The model under review builds one solid part; all positions refer to its coordinate system, in mm. A direction names the side the tool comes from. Round coordinates to 2 decimals unless told otherwise and drop trailing zeros. Write each loop counter-clockwise with the first axis right and the second up, starting at its lowest first coordinate (ties: lowest second). Pieces come first, ordered by that corner, then holes. Notation, with made-up numbers: (65.5, 20) -> (70.5, 20) arc R17 ccw to (70.5, 27) -> close; hole circle Ø2 at (70.25, 18.5). An arc over 180 degrees is marked (long way). Answer as a JSON object with one key per item and string values. Group by question number.
1) We need section A-A, the plane y = 11.5. Write out the cut boundary in (x, z) (1 decimal).
2) Machinability: for faces 1 (the flat face through (4, 0, 0)), 2 (the flat face through (-4, 17.78, 0)), 3 (the cylindrical face through (-8.68, 29.77, 1.93)), which of the approach directions +Z, -Z, +X, -X, +Y, -Y give a long, thin tool a straight path to every point of the face, cutting with its end or side? Answer none if there is none.
3) We need section C-C, the plane x = 4. Write out the cut boundary in (y, z) (3 decimals).
4) We need section B-B, the plane z = 6.5. Write out the cut boundary in (x, y) (3 decimals).
5) Mouldability with a two-part tool opening along X and no side actions: class faces 4 (the cylindrical face through (0.708, 28.486, 3.186)), 5 (the cylindrical face through (7.5, 15, -8.2)), 6 (the flat face through (9.1, 24.765, 0.1)) as pulls with the +X half, pulls with the -X half, needs draft (parallel to the pull), parting line crosses it, or undercut.
6) We need section D-D, the plane x = -8. Write out the cut boundary in (y, z) (3 decimals), then the cut area to 3 significant figures.
7) To check wall thickness, follow probe 1 along Y at (x, z) = (4, 0) (3 decimals); probe 2 along Y at (x, z) = (-6.5, -7.5) (3 decimals); probe 3 along Z at (x, y) = (5.5, 8.89). State the ranges of each line that lie inside material, in increasing order. Write a range as [from, to].
8) Insertion check: pin 1 Ø1.5 at (y, z) = (4.5, -9) entering from +X; pin 2 Ø8 at (y, z) = (6, 3.5) entering from +X; pin 3 Ø2 at (y, z) = (28, -1.5) entering from +X. Each pin has a flat end and moves straight along its axis. Give the tip position at first contact, or say it passes through.
from build123d import *

# Parameters (mm, degrees)
CROQUIS1_R                     = 11.1125
SALIENTE_EXTRUIR1_DEPTH        = 34.925
CORTAR_EXTRUIR2_START          = 10.16
CROQUIS12_R                    = 11.1125
CROQUIS12_R_2                  = 8.89
CORTAR_EXTRUIR2_DEPTH          = 10.16
TALADRO_ROSCADO_5_16_181_D     = 6.5278
TALADRO_ROSCADO_5_16_181_DEPTH = 12.7
TALADRO_ROSCADO_5_16_181_TIP   = 1.961148974
CROQUIS6_W                     = 22.225
CROQUIS6_H                     = 17.78
CORTAR_EXTRUIR1_DEPTH          = 25.4
TALADRO_ROSCADO_5_8_181_D      = 14.68374
TALADRO_ROSCADO_5_8_181_DEPTH  = 38.7985
TALADRO_ROSCADO_5_8_181_TIP    = 4.411440553


with BuildPart() as part:
    # Croquis1 → Saliente-Extruir1 (new body)
    with BuildSketch(Plane(origin=(0, 0, 0), x_dir=(1, 0, 0), z_dir=(0, 1, 0))):
        with Locations(Location((0, 0, 0), (0, 0, 270))):
            Circle(CROQUIS1_R)
    extrude(amount=SALIENTE_EXTRUIR1_DEPTH)

    # Croquis12 → Cortar-Extruir2 (cut)
    with BuildSketch(Plane.XZ.offset(-34.925).offset(CORTAR_EXTRUIR2_START)):
        with Locations(Location((0, 0, 0), (0, 0, 270))):
            Circle(CROQUIS12_R)
        with Locations(Location((0, 0, 0), (0, 0, 270))):
            Circle(CROQUIS12_R_2, mode=Mode.SUBTRACT)
    extrude(amount=-CORTAR_EXTRUIR2_DEPTH, mode=Mode.SUBTRACT)

    # Taladro roscado 5/16-181
    with Locations(Plane(origin=(0, 34.925, 0), x_dir=(1, 0, 0), z_dir=(0, 1, 0))):
        with Locations((0, 0)):
            Hole(TALADRO_ROSCADO_5_16_181_D / 2, depth=TALADRO_ROSCADO_5_16_181_DEPTH)
            with Locations((0, 0, -(TALADRO_ROSCADO_5_16_181_DEPTH + TALADRO_ROSCADO_5_16_181_TIP / 2))):  # 118° drill point
                Cone(0, TALADRO_ROSCADO_5_16_181_D / 2, TALADRO_ROSCADO_5_16_181_TIP, mode=Mode.SUBTRACT)

    # Croquis6 → Cortar-Extruir1 (cut)
    with BuildSketch(Plane(origin=(0, 0, 0), x_dir=(0, 0, -1), z_dir=(1, 0, 0))):
        with Locations((0, 8.89)):
            Rectangle(CROQUIS6_W, CROQUIS6_H)
    extrude(amount=-CORTAR_EXTRUIR1_DEPTH, mode=Mode.SUBTRACT)

    # Taladro roscado 5/8-181
    with Locations(Plane.ZY):
        with Locations((0, 8.89)):
            Hole(TALADRO_ROSCADO_5_8_181_D / 2, depth=TALADRO_ROSCADO_5_8_181_DEPTH)
            with Locations((0, 0, -(TALADRO_ROSCADO_5_8_181_DEPTH + TALADRO_ROSCADO_5_8_181_TIP / 2))):  # 118° drill point
                Cone(0, TALADRO_ROSCADO_5_8_181_D / 2, TALADRO_ROSCADO_5_8_181_TIP, mode=Mode.SUBTRACT)


solid = part.part
Here are the results:
{
 "1": {"outline": "(0, -11.1) arc R11.1 ccw to (8.7, -6.9) -> (0, -6.9) -> close; (0, 6.9) -> (8.7, 6.9) arc R11.1 ccw to (0, 11.1) -> close"},
 "2": {"face 1": "+Z, -Z, +X, -X, -Y", "face 2": "+Z, -Z, -X, -Y", "face 3": "+Y"},
 "3": {"outline": "(0, -10.368) -> (24.765, -10.368) -> (24.765, -7.939) -> (34.925, -7.939) -> (34.925, 7.939) -> (24.765, 7.939) -> (24.765, 10.368) -> (0, 10.368) -> close; hole circle Ø14.684 at (8.89, 0)"},
 "4": {"outline": "(-9.013, 17.78) -> (0, 17.78) -> (0, 12.304) -> (9.013, 12.304) -> (9.013, 24.765) -> (6.065, 24.765) -> (6.065, 34.925) -> (-6.065, 34.925) -> (-6.065, 24.765) -> (-9.013, 24.765) -> close; (0, 0) -> (9.013, 0) -> (9.013, 5.476) -> (0, 5.476) -> close"},
 "5": {"face 4": "undercut", "face 5": "parting line crosses it", "face 6": "needs draft"},
 "6": {"outline": "(17.78, -7.713) -> (24.765, -7.713) -> (24.765, -3.877) -> (34.925, -3.877) -> (34.925, 3.877) -> (24.765, 3.877) -> (24.765, 7.713) -> (17.78, 7.713) -> close", "area": "187 mm^2"},
 "7": {"probe 1": "y = [0, 1.548], [16.232, 34.925]", "probe 2": "y = [17.78, 24.765]", "probe 3": "z = [-9.66, -7.34], [7.34, 9.66]"},
 "8": {"pin 1": "stops at x = 7.44", "pin 2": "stops at x = 10.77", "pin 3": "stops at x = 8.88"}
}
